```python
from build123d import *

# Parameters (mm, degrees)
F0_W     = 482.6
F0_H     = 114.3
F0_R     = 2.921
F0_R_2   = 2.032
F0_W_2   = 47.498
F0_H_2   = 27.686
F1_DEPTH = 2.286


with BuildPart() as f1:
    # F0 (on Front) → F1 (new body)
    with BuildSketch(Plane.XZ):
        with Locations((157.3911, 0)):
            Rectangle(F0_W, F0_H)
        with Locations((-33.1089, -41.3258)):
            Circle(F0_R, mode=Mode.SUBTRACT)
        with Locations((33.1089, -41.3258)):
            Circle(F0_R, mode=Mode.SUBTRACT)
        with Locations((0, -19.939)):
            Circle(F0_R_2, mode=Mode.SUBTRACT)
        Rectangle(F0_W_2, F0_H_2, mode=Mode.SUBTRACT)
        with Locations((0, 19.939)):
            Circle(F0_R_2, mode=Mode.SUBTRACT)
        with Locations((-33.1089, 41.3258)):
            Circle(F0_R, mode=Mode.SUBTRACT)
        with Locations((33.1089, 41.3258)):
            Circle(F0_R, mode=Mode.SUBTRACT)
    extrude(amount=F1_DEPTH)


solid = f1.part
```
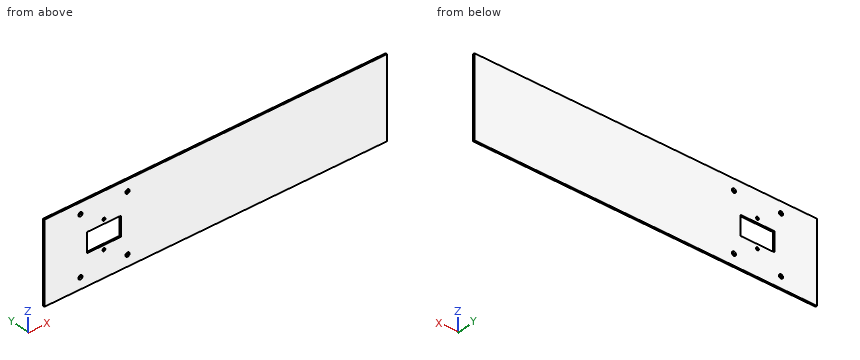
Build history of the part. All positions in model axes, mm. Round coordinates to 2 decimals unless told otherwise and drop trailing zeros. Loops run counter-clockwise (first coordinate to the right, second up) from the corner with the lowest first, then second, coordinate; pieces in that order, holes last.
Item 1: Drill centre lines: line 1 along X through (y, z) = (-2.15, -1); line 2 along Z through (x, y) = (0, -0.65); line 3 along X through (y, z) = (-1, -42.5). Where is each one in solid material? Low to high.
Item 2: Saw through at A-A (y = -0.6). List the corners of the cut face in (x, z), then the cut area to 3 significant figures.
Item 3: Pin check, flat tip, straight feed: P1, Ø4.5, axis at x = -33.11, z = 41.33, coming from the -Y side. Stop position of the tip, or through.
Worked answers:
1. line 1: x = -83.91 to -23.75, 23.75 to 398.69
1. line 2: z = -57.15 to -21.97, -17.91 to -13.84, 13.84 to 17.91, 21.97 to 57.15
1. line 3: x = -83.91 to -35.78, -30.43 to 30.43, 35.78 to 398.69
2. outline: (-83.91, -57.15) - (398.69, -57.15) - (398.69, 57.15) - (-83.91, 57.15) - close; hole circle Ø5.84 at (-33.11, -41.33); hole circle Ø5.84 at (-33.11, 41.33); hole (-23.75, -13.84) - (23.75, -13.84) - (23.75, 13.84) - (-23.75, 13.84) - close; hole circle Ø4.06 at (0, -19.94); hole circle Ø4.06 at (0, 19.94); hole circle Ø5.84 at (33.11, -41.33); hole circle Ø5.84 at (33.11, 41.33)
2. area: 53,700 mm2
3. P1: passes through
